Check sheet for the modelled part. Datum: model origin and axes. Units: mm. Face numbers are marked on the shaded views. Give positions to 0.01 mm unless a question says otherwise; leave off trailing zeros. Order: outer loops, then holes, each group sorted by start corner. A loop starts at its lowest first (then second) coordinate and runs counter-clockwise, first axis right, second up. Notation, with made-up numbers: M 74,22.25 L 125,22.25 A19 cw 125,47.25 Z; hole C 25,-19.5 d3. An arc over 180 degrees is marked long. Return JSON: item names as keys, results as strings. Group by question number.
Autodesk Fusion 360 part; units mm, degrees
sketch "スケッチ1" plane through (0, 0, 0) normal (0, 0, 1) x (1, 0, 0)
  line L0 (-4, -4) -> (10, -4)
  line L1 (10, -4) -> (12.5, -1.5)
  line L2 (12.5, -1.5) -> (19, -1.5)
  line L3 (19, -1.5) -> (19, 4)
  line L4 (19, 4) -> (-4, 4)
  line L5 (-4, 4) -> (-4, -4)
  line L6 (-4, 0) -> (0, 0) construction
  circle A0 centre (0, 0) radius 1.5
  circle A1 centre (0, 0) radius 2.5
  dimension "d1" = 23
  dimension "d2" = 8
  dimension "d3" = 5.5
  dimension "d4" = 14
  dimension "d5" = 45
  dimension "d6" = 4
  dimension "d7" = 3
  dimension "d8" = 5
extrude "押し出し1" add sketch "スケッチ1" along normal blind 1.6 contours L0 L1 L2 L3 L4 L5
extrude "押し出し2" add sketch "スケッチ1" along normal blind 2 contours A1
fillet "フィレット1" radius 1 4 edges at (-4, 4, 0.8) (19, 4, 0.8) (19, -1.5, 0.8) (-4, -4, 0.8)
fillet "フィレット2" radius 0.5 2 edges at (12.5, -1.5, 0.8) (10, -4, 0.8)
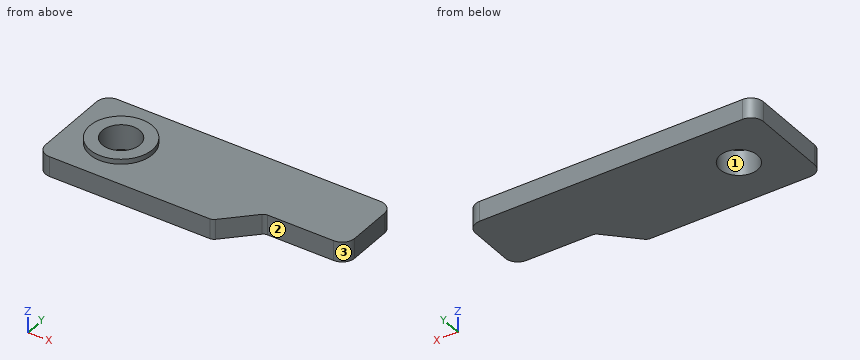
1) Material ranges on line 1 along Y through (x, z) = (0, 0.4); line 2 along Z through (x, y) = (7.75, 2.75); line 3 along Y through (x, z) = (17, 1.15), recorded low to high.
2) Depth check by flat-ended pin: P1, Ø2.5, axis at x = 0, y = 0, coming from the +Z side. Enter the tip coordinate at first touch or a pass-through.
3) Sectioned sample at A-A on y = 0. Record the boundary of the cut face in (x, z).
4) Sectioned sample at B-B on z = 1. Record the boundary of the cut face in (x, y), then the cut area to 3 significant figures.
5) Release check for a two-part mould opening along X. For the marked faces 1, 2 and 3 record: released by +X, released by -X, zero draft, split by the parting line, or undercut.
6) Sectioned sample at D-D on y = -2. Record the boundary of the cut face in (x, z).
7) Sectioned sample at C-C on x = 0. Record the boundary of the cut face in (y, z), then the cut area to 3 significant figures.
Reply:
{
 "1": {"line 1": "-4 to -1.5, 1.5 to 4", "line 2": "0 to 1.6", "line 3": "-1.5 to 4"},
 "2": {"P1": "through"},
 "3": {"outline": "M -4,0 L -1.5,0 L -1.5,2 L -2.5,2 L -2.5,1.6 L -4,1.6 Z; M 1.5,0 L 19,0 L 19,1.6 L 2.5,1.6 L 2.5,2 L 1.5,2 Z"},
 "4": {"outline": "M -4,-3 A1 ccw -3,-4 L 9.79,-4 A0.5 ccw 10.15,-3.85 L 12.35,-1.65 A0.5 cw 12.71,-1.5 L 18,-1.5 A1 ccw 19,-0.5 L 19,3 A1 ccw 18,4 L -3,4 A1 ccw -4,3 Z; hole C 0,0 d3", "area": "157 mm^2"},
 "5": {"face 1": "undercut", "face 2": "zero draft", "face 3": "released by +X"},
 "6": {"outline": "M -4,0 L 12,0 L 12,1.6 L 1.5,1.6 L 1.5,2 L -1.5,2 L -1.5,1.6 L -4,1.6 Z"},
 "7": {"outline": "M -4,0 L -1.5,0 L -1.5,2 L -2.5,2 L -2.5,1.6 L -4,1.6 Z; M 1.5,0 L 4,0 L 4,1.6 L 2.5,1.6 L 2.5,2 L 1.5,2 Z", "area": "8.80 mm^2"}
}
